Geometry check sheet. Reference: drawing and pictorial views, mm from the part's lowest x, y, z. Give positions to 0.01 mm unless a question says otherwise; leave off trailing zeros. Order: outer loops, then holes, each group sorted by start corner. A loop starts at its lowest first (then second) coordinate and runs counter-clockwise, first axis right, second up.
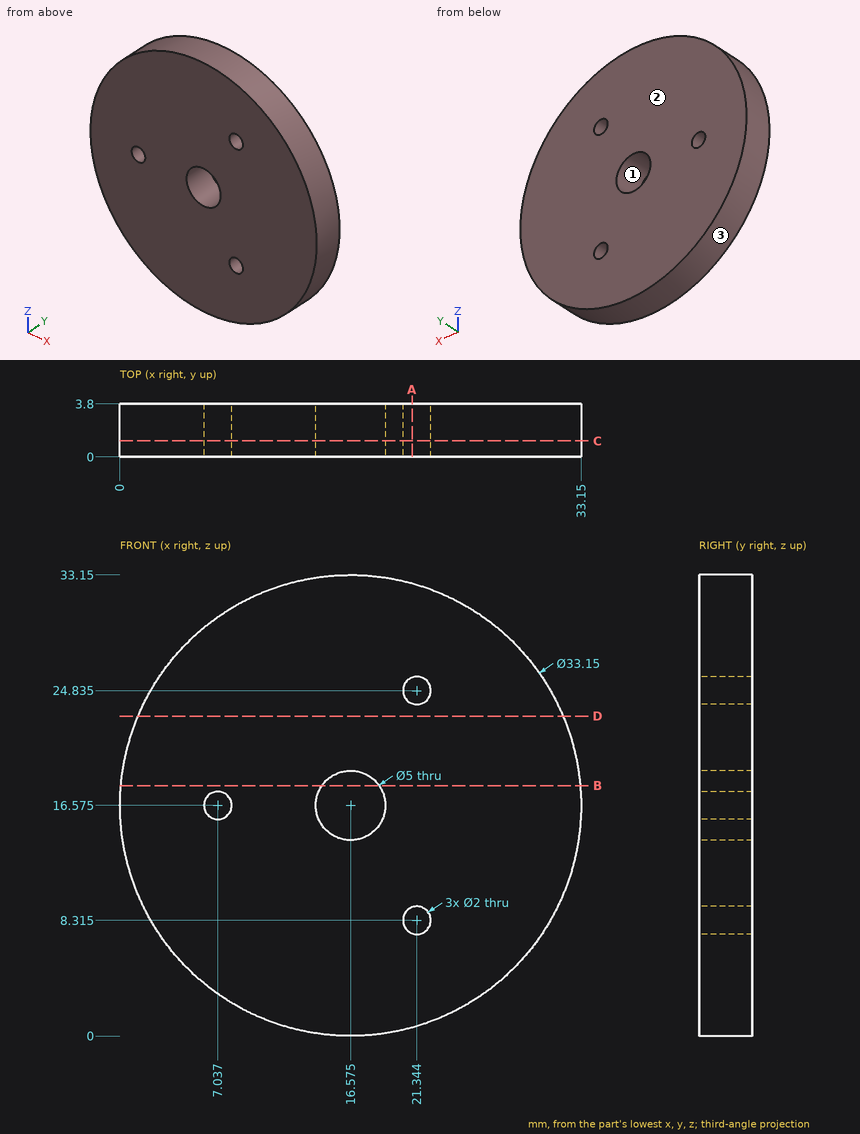
(1) Sectioned sample at B-B (z = 18). Enter the section's corners in (x, y), plus the area to 3 significant figures.
(2) Sectioned sample at C-C (y = 1.15). Count the separate pieces of the cut face and the enclosed holes in it, plus the area to 3 significant figures.
(3) Release check for a two-part mould opening along Z. For the marked faces 1, 2 and 3 record: released by +Z, released by -Z, zero draft, split by the parting line, or undercut.
(4) Sectioned sample at D-D (z = 23). Enter the section's corners in (x, y) (1 decimal).
(5) Sectioned sample at A-A (x = 21). Enter the section's corners in (y, z) (1 decimal), plus the area to 3 significant figures.
(6) Go/stop test with flat-tipped pins: P1, Ø2, axis at x = 6.5, y = 2.5, coming from the -Z side (1 decimal); P2, Ø1.8, axis at x = 21.34, z = 8.32, coming from the +Y side; P3, Ø2, axis at x = 14.5, y = 3, coming from the +Z side (1 decimal). Record where each tip stops, or that it passes through.
(7) Thickness scan on L1, parallel to Z at x = 16.5, y = 0.4; L2, parallel to Z at x = 21.5, y = 3; L3, parallel to X at y = 0.8, z = 17 (1 decimal). Record the ranges inside material, lowest first.
Values follow:
1. outline: (0.06, 0) - (14.52, 0) - (14.52, 3.8) - (0.06, 3.8) - close; (18.63, 0) - (33.09, 0) - (33.09, 3.8) - (18.63, 3.8) - close
1. area: 110 mm2
2. separate pieces: 1
2. enclosed holes: 4
2. area: 834 mm2
3. face 1: undercut
3. face 2: zero draft
3. face 3: split by the parting line
4. outline: (1.3, 0) - (31.9, 0) - (31.9, 3.8) - (1.3, 3.8) - close
5. outline: (0, 0.6) - (3.8, 0.6) - (3.8, 7.4) - (0, 7.4) - close; (0, 9.3) - (3.8, 9.3) - (3.8, 23.9) - (0, 23.9) - close; (0, 25.8) - (3.8, 25.8) - (3.8, 32.5) - (0, 32.5) - close
5. area: 107 mm2
6. P1: stops at z = 2.7
6. P2: passes through
6. P3: stops at z = 33.1
7. L1: z = 0 to 14.08, 19.07 to 33.15
7. L2: z = 0.75 to 7.33, 9.3 to 23.85, 25.82 to 32.4
7. L3: x = 0 to 6.1, 7.9 to 14.1, 19 to 33.1
